For this review, take the finished solid that the model builds, in its own axes (mm). Face numbers are marked on the shaded views. A direction names the side the tool comes from. Give positions to 0.01 mm unless a question says otherwise; leave off trailing zeros. Loops run counter-clockwise (first coordinate to the right, second up) from the corner with the lowest first, then second, coordinate; pieces in that order, holes last. Notation, with made-up numbers: (78.25, -31) -> (90.25, -31) arc R31 cw to (90.25, -6) -> close; hole circle Ø7 at (-13.5, -36.75). An arc over 180 degrees is marked (long way). One line per question, with ' | ' between items. Start each with the question number.
(1) Consider section A-A (z = -15). Give the number of separate pieces and of enclosed holes in the cut face, and give its area (3 significant figures).
(2) Insertion check: P1, Ø22, axis at x = 10.5, y = 9.5, coming from the +Z side; P2, Ø8, axis at y = 75.5, z = -24, coming from the -X side; P3, Ø5, axis at x = 10, z = -3.5, coming from the -Y side. Each pin has a flat end and moves straight along its axis. Give the tip position at first contact, or say it passes through.
(3) Tool access review of the marked faces 5, 6, 7, 8 and 9: name each direction out of +Z, -Z, +X, -X, +Y, -Y from which nothing blocks a thin tool from reaching the whole face with its end or side.
(4) Consider section B-B (y = 6.56). Write out the cut boundary in (x, z).
(5) Draft analysis for pull direction Y (two halves, no side actions). For the marked faces 1, 2, 3 and 4, state which applies: +Y half, -Y half, draft (parallel to the pull), parting line (faces both ways), or undercut.
(6) Wall thickness on probe 1 along Y at (x, z) = (21.6, -15) (1 decimal); probe 2 along Z at (x, y) = (28.5, 6.56); probe 3 along Y at (x, z) = (28.5, -15) (3 decimals): over which ranges is each line inside the solid? List them lowest first.
(7) Consider section C-C (x = 1.5). Write out the cut boundary in (y, z).
(8) Consider section D-D (y = 68). Write out the cut boundary in (x, z), and give its area (3 significant figures).
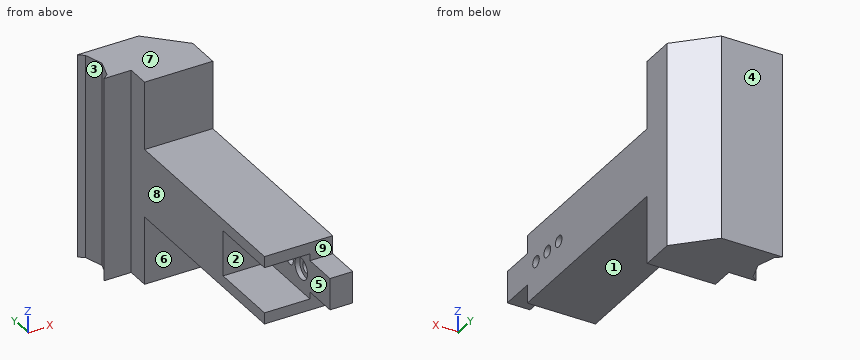
Autodesk Inventor part; units mm, degrees
ref_plane "Work Plane1" through (0, 0, -15) normal (0, 0, 1) x (1, 0, 0)
ref_plane "YZ Plane" through (0, 0, 0) normal (1, 0, 0) x (0, 1, 0)
ref_plane "XZ Plane" through (0, 0, 0) normal (0, 1, 0) x (-1, 0, 0)
sketch "Sketch1" plane through (0, 0, 0) normal (0, 0, 1) x (1, 0, 0)
  line L0 (0, 0) -> (25, 0)
  line L1 (25, 0) -> (25, 40)
  line L2 (25, 40) -> (0, 40)
  line L3 (0, 40) -> (0, 0)
  dimension "d1" = 25
  dimension "d2" = 40
  dimension "d3" = 25
extrude "Extrusion1" add sketch "Sketch1" against normal blind 30
sketch "Sketch2" plane through (25, 0, 0) normal (1, 0, 0) x (0, 0, -1)
  line L0 (0, 0) -> (30, 0)
  circle A0 centre (15, 6.56) radius 2.46
extrude "Extrusion2" cut sketch "Sketch2" against normal blind 30
sketch "Sketch3" plane through (0, 0, 0) normal (-1, 0, 0) x (0, 0, 1)
  line L0 (0, 0) -> (-30, 0)
  line L1 (-25.05, 0) -> (-4.95, 0)
  line L2 (-4.95, 0) -> (-4.95, 33.12)
  line L3 (-4.95, 33.12) -> (-25.05, 33.12)
  line L4 (-25.05, 33.12) -> (-25.05, 0)
  dimension "d11" = 20.1
extrude "Extrusion3" cut sketch "Sketch3" against normal blind 20
sketch "Sketch4" plane through (0, 0, 0) normal (0, -1, 0) x (1, 0, 0)
  line L0 (20, -4.95) -> (20, -25.05)
  line L1 (20, -15) -> (25, -15)
  line L2 (25, 0) -> (25, -30)
  line L3 (20, -8.025) -> (25, -8.025)
  line L4 (25, -8.025) -> (25, -21.975)
  line L5 (25, -21.975) -> (20, -21.975)
  line L6 (20, -21.975) -> (20, -8.025)
  line L7 (20, -8.025) -> (25, -21.975) construction
  line L8 (25, -8.025) -> (20, -21.975) construction
  line L9 (25, -12.54) -> (25, -17.46)
  point P0 (0, 0)
  point P1 (22.5, -15)
  dimension "d14" = 13.95
extrude "Extrusion4" add sketch "Sketch4" along normal blind 15
sketch "Sketch5" plane through (20, 0, 0) normal (-1, 0, 0) x (0, 0, 1)
  circle A0 centre (-15, 6.56) radius 2.46
  circle A1 centre (-15, 6.56) radius 4.7025
  circle A2 centre (-15, 6.56) radius 2.46
  circle A3 centre (-15, 6.56) radius 2.46
  point P0 (0, 0)
  dimension "d17" = 9.405
extrude "Extrusion5" cut sketch "Sketch5" against normal blind 2.1
sketch "Sketch6" plane through (25, 0, 0) normal (1, 0, 0) x (0, 0, -1)
  circle A0 centre (15, 6.56) radius 4.7025
  line L0 (15, 6.56) -> (15, 23.56)
  circle A1 centre (15, 23.56) radius 2.46
  point P0 (0, 0)
  dimension "d20" = 17
  dimension "d21" = 4.92
extrude "Extrusion6" cut sketch "Sketch6" against normal blind 10 contours A1
sketch "Sketch7" plane through (20, 0, 0) normal (-1, 0, 0) x (0, 0, 1)
  circle A0 centre (-15, 23.56) radius 2.46
  circle A1 centre (-15, 23.56) radius 4.7025
  point P0 (0, 0)
  dimension "d24" = 9.405
extrude "Extrusion7" cut sketch "Sketch7" against normal blind 2.1
sketch "Sketch9" plane through (25, 0, 0) normal (1, 0, 0) x (0, 0, -1)
  circle A0 centre (15, 6.56) radius 2.46
  circle A1 centre (15, 6.56) radius 2.46
  circle A2 centre (15, 23.56) radius 2.46
  circle A3 centre (15, 23.56) radius 2.46
  line L0 (30, 40) -> (30, 0)
  line L1 (30, 0) -> (30, 40)
  line L2 (30, 40) -> (0, 40)
  line L3 (0, 40) -> (0, 0)
  line L4 (0, 0) -> (8.025, 0)
  line L5 (21.975, 0) -> (21.975, -15)
  line L6 (21.975, -15) -> (8.025, -15)
  line L7 (8.025, -15) -> (8.025, 0)
  line L8 (0, 0) -> (8.025, 0)
  line L9 (21.975, 0) -> (30, 0)
extrude "Extrusion8" add sketch "Sketch9" along normal blind 5
sketch "Sketch10" plane through (0, 40, 0) normal (0, 1, 0) x (1, 0, 0)
  line L0 (0, 30) -> (30, 30)
  line L1 (30, 0) -> (0, 0)
  line L2 (0, 30) -> (30, 30)
  line L3 (30, 30) -> (30, 0)
  line L4 (30, 0) -> (0, 0)
  line L5 (0, 0) -> (0, 30)
extrude "Extrusion9" add sketch "Sketch10" along normal blind 30
sketch "Sketch12" plane through (30, 0, 0) normal (1, 0, 0) x (0, 0, -1)
  circle A0 centre (15, 6.56) radius 2.46
  line L0 (15, 6.56) -> (15, 15.06)
  circle A1 centre (15, 15.06) radius 2.525
  point P0 (0, 0)
  dimension "d31" = 8.5
  dimension "d33" = 5.05
extrude "Extrusion10" cut sketch "Sketch12" against normal blind 30 contours A1
sketch "Sketch14" plane through (0, 0, 0) normal (0, 0, 1) x (1, 0, 0)
  line L0 (30, 70) -> (0, 70)
  line L1 (0, 70) -> (0, 85)
  line L2 (30, 0) -> (30, 70)
  line L3 (30, 100) -> (30, 70)
  line L4 (-12, 120) -> (15, 120)
  line L5 (-9.5, 118) -> (-7, 110)
  line L6 (-9.5, 118) -> (-12, 120)
  line L7 (-9.5, 102) -> (-7, 110)
  line L8 (-9.5, 102) -> (-12, 100)
  line L9 (30, 105) -> (15, 120)
  line L10 (30, 105) -> (30, 100)
  line L11 (0, 85) -> (0, 100)
  line L12 (0, 100) -> (-12, 100)
  point P0 (0, 0)
  dimension "d60" = 20
  dimension "d64" = 12
extrude "Extrusion12" add sketch "Sketch14" against normal blind 30
sketch "Sketch15" plane through (0, 0, -25.05) normal (-1, 0, 0) x (0, 0, 1)
  line L0 (0, 33.12) -> (20.1, 33.12)
  line L1 (20.1, 33.12) -> (20.1, 0)
  line L2 (0, 33.12) -> (20.1, 33.12)
  line L3 (20.1, 33.12) -> (20.1, 31.1)
  line L4 (20.1, 31.1) -> (0, 31.1)
  line L5 (0, 31.1) -> (0, 33.12)
  point P0 (25.05, 0)
  dimension "d57" = 2.02
extrude "Extrusion13" add sketch "Sketch15" against normal blind 20
sketch "Sketch20" plane through (0, 0, 0) normal (0, 0, 1) x (1, 0, 0)
  line L0 (0, 100) -> (-12, 100)
  line L1 (0, 100) -> (-12, 100)
  line L2 (-12, 100) -> (-9.5, 102)
  line L3 (-12, 100) -> (-9.5, 102)
  line L4 (-9.5, 102) -> (-7, 110)
  line L5 (-9.5, 102) -> (-7, 110)
  line L6 (-7, 110) -> (-9.5, 118)
  line L7 (-7, 110) -> (-9.5, 118)
  line L8 (-9.5, 118) -> (-12, 120)
  line L9 (-9.5, 118) -> (-12, 120)
  line L10 (-12, 120) -> (15, 120)
  line L11 (-12, 120) -> (15, 120)
  line L12 (15, 120) -> (30, 105)
  line L13 (15, 120) -> (30, 105)
  line L14 (30, 105) -> (30, 90)
  line L15 (30, 0) -> (30, 105)
  line L16 (30, 90) -> (0, 90)
  line L17 (0, 90) -> (0, 100)
  point P0 (0, 0)
  dimension "d65" = 15
  dimension "d66" = 30
extrude "Extrusion14" add sketch "Sketch20" along normal blind 30
ref_plane "Work Plane1" through (0, 0, -15) normal (0, 0, 1) x (1, 0, 0)
mirror "Mirror1" about plane through (0, 0, -15) normal (0, 0, 1) of "Extrusion14"
properties part number "rec_b_16mm_x_90mm"
A:
1) separate pieces: 4 | enclosed holes: 0 | area: 3,020 mm^2
2) P1: stops at z = 0 | P2: stops at x = 0 | P3: stops at y = 0
3) face 5: -X, -Y | face 6: -Z, +X, -X, -Y | face 7: +Z, +X, -X, +Y, -Y | face 8: +Z, -Z, -X, -Y | face 9: +Z, +X, -X, -Y
4) outline: (0, -30) -> (30, -30) -> (30, -17.46) -> (22.1, -17.46) -> (22.1, -19.7) -> (20, -19.7) -> (20, -25.05) -> (0, -25.05) -> close; (0, -4.95) -> (20, -4.95) -> (20, -10.3) -> (22.1, -10.3) -> (22.1, -12.54) -> (30, -12.54) -> (30, 0) -> (0, 0) -> close
5) face 1: draft | face 2: -Y half | face 3: undercut | face 4: +Y half
6) probe 1: y = -15 to 1.9, 11.3 to 12.5, 17.6 to 18.9, 28.3 to 113.4 | probe 2: z = -30 to -17.46, -12.54 to 0 | probe 3: y = -15 to 4.1, 9.02 to 12.535, 17.585 to 21.1, 26.02 to 106.5
7) outline: (0, -30) -> (90, -30) -> (90, -60) -> (120, -60) -> (120, 30) -> (90, 30) -> (90, 0) -> (0, 0) -> (0, -4.95) -> (31.1, -4.95) -> (31.1, -25.05) -> (0, -25.05) -> close
8) outline: (0, -30) -> (30, -30) -> (30, 0) -> (0, 0) -> close | area: 900 mm^2
